Can you work these out from the model? Positions are in its coordinate system, mm. Face numbers are marked on the shaded views. A direction names the side the tool comes from. Coordinates: 2 decimals unless noted, no trailing zeros. Loops run counter-clockwise (first coordinate to the right, second up) from the corner with the lowest first, then second, coordinate; pieces in that order, holes last. Notation, with made-up numbers: (3, -4) - (40, -4) arc R10 cw to (40, 5) - close; hole circle Ø5 at (-11.75, 36). An arc over 180 degrees is marked (long way). Put each result on its own line as item: value. Start each with the question number.
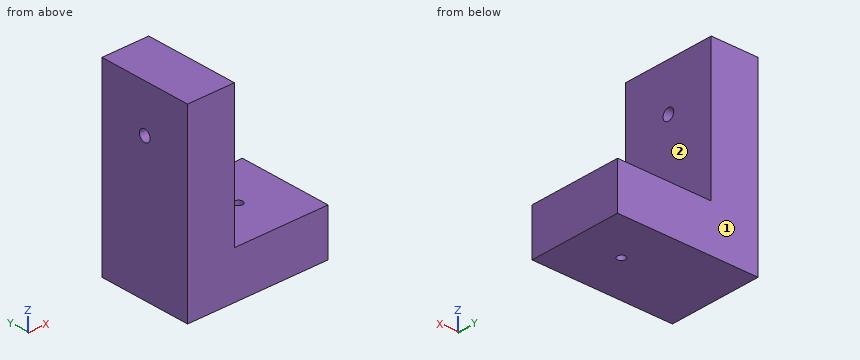
from build123d import *

# Parameters (mm, degrees)
F1_DEPTH = 101.6
F4_DEPTH = 115.900189
F5_DEPTH = 182.793036


with BuildPart() as f1:
    # F0 (on Front) → F1 (new body)
    with BuildSketch(Plane.XZ):
        Polygon((50.8, 101.044822), (0, 101.044822), (0, -102.155178), (152.4, -102.155178), (152.4, -51.355178), (50.8, -51.355178), align=None)
    extrude(amount=F1_DEPTH)

    # F3 (on face) → F4 (cut)
    with BuildSketch(Plane.XY.offset(-51.355178)):
        with BuildLine():
            ThreePointArc((106.1085, -50.8), (101.6, -46.2915), (97.0915, -50.8))
            ThreePointArc((97.0915, -50.8), (101.6, -55.3085), (106.1085, -50.8))
        make_face()
    extrude(amount=-F4_DEPTH, mode=Mode.SUBTRACT)

    # F2 (on face) → F5 (cut)
    with BuildSketch(Plane.YZ.offset(50.8)):
        with BuildLine():
            ThreePointArc((-44.45, 50.244822), (-46.309872, 54.73495), (-50.8, 56.594822))
            ThreePointArc((-50.8, 56.594822), (-55.290128, 45.754694), (-44.45, 50.244822))
        make_face()
    extrude(amount=-F5_DEPTH, mode=Mode.SUBTRACT)


solid = f1.part
Q1. On a 3-axis mill with a long thin cutter (end or side, diameter ignored), from which of +Z, -Z, +X, -X, +Y, -Y can I reach the whole of each face in a straight line? I mean the marked faces 1 and 2. Say none if no direction works.
Q2. Please list where these lines run through material, in increasing order: line 1 along X through (y, z) = (-50.8, -88.5); line 2 along Z through (x, y) = (59.5, -19.5); line 3 along X through (y, z) = (-73, 0). Write a range as [from, to].
Q3. Will these pins go through, and if not, where does the flat tip stop? pin 1 (10 mm diameter, centred on y = -64.5, z = -28.5, fed in from +X); pin 2 (11.5 mm diameter, centred on y = -50.8, z = 50.24, fed in from +X); pin 3 (1.5 mm diameter, centred on y = -88, z = -61.5, fed in from -X).
Q4. I want a section at C-C on z = 1. List the corners of the cut face in (x, y) for me.
Q5. I want a section at D-D on x = 67. List the corners of the cut face in (y, z) for me, and give its area (3 significant figures).
Q6. I want a section at B-B on y = -11. List the corners of the cut face in (x, z) for me.
Q7. I want a section at A-A on x = 101.6. List the corners of the cut face in (y, z) for me, and give its area (3 significant figures).
Calculated:
1. face 1: +Z, -Z, +X, -X, +Y
1. face 2: +Z, +X, +Y, -Y
2. line 1: [0, 97.09], [106.11, 152.4]
2. line 2: [-102.16, -51.36]
2. line 3: [0, 50.8]
3. pin 1: x = 50.8
3. pin 2: through
3. pin 3: x = 0
4. outline: (0, -101.6) - (50.8, -101.6) - (50.8, 0) - (0, 0) - close
5. outline: (-101.6, -102.16) - (0, -102.16) - (0, -51.36) - (-101.6, -51.36) - close
5. area: 5,160 mm2
6. outline: (0, -102.16) - (152.4, -102.16) - (152.4, -51.36) - (50.8, -51.36) - (50.8, 101.04) - (0, 101.04) - close
7. outline: (-101.6, -102.16) - (-55.31, -102.16) - (-55.31, -51.36) - (-101.6, -51.36) - close; (-46.29, -102.16) - (0, -102.16) - (0, -51.36) - (-46.29, -51.36) - close
7. area: 4,700 mm2
